Input: dimensioned drawing with shaded views. Units: mm. Origin: part minimum x, y, z. Round coordinates to 2 decimals unless told otherwise and drop trailing zeros. Write each loop counter-clockwise with the first axis right and the second up, starting at its lowest first coordinate (ties: lowest second). Pieces come first, ordered by that corner, then holes. Notation, with made-up numbers: (48, 53.25) - (105, 53.25) arc R31 cw to (105, 91.25) - close; hole circle Ø8 at (75, 69). An arc over 180 degrees is marked (long way). Use one line per item in the form item = value.
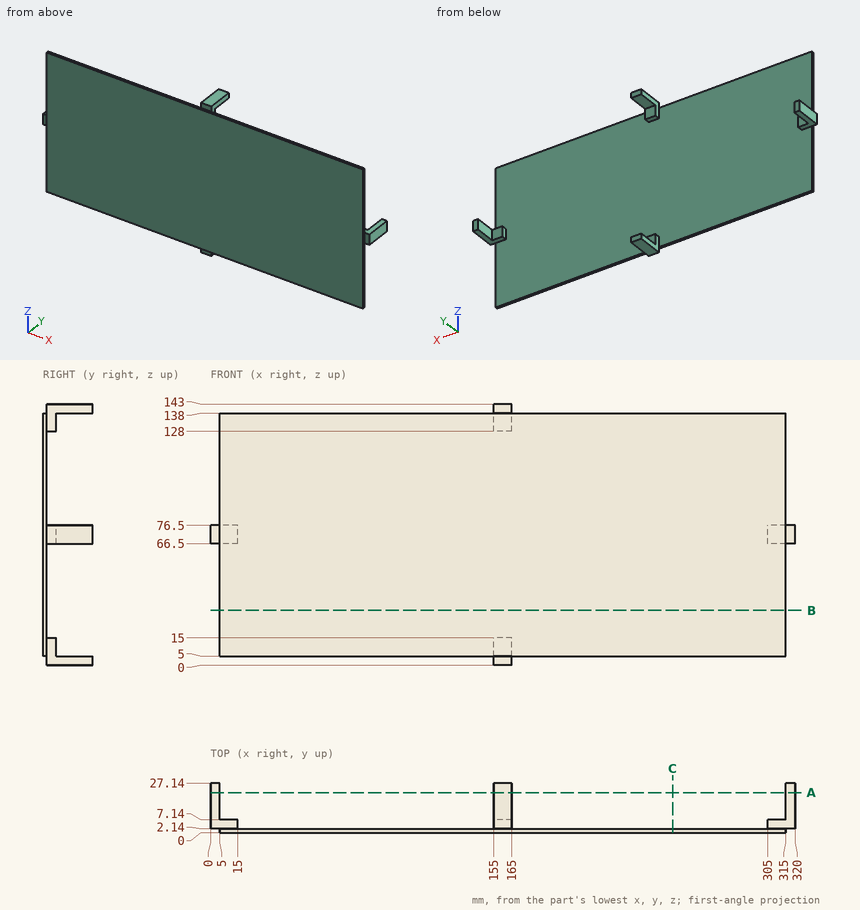
(1) Cut plane B-B on z = 30. Output: boundary loops of the cut face in (x, y).
Derived:
outline = (5, 0) - (315, 0) - (315, 2.14) - (5, 2.14) - close
(2) Cut plane C-C on x = 253. Output: boundary loops of the cut face in (y, z).
Derived:
outline = (0, 5) - (2.14, 5) - (2.14, 138) - (0, 138) - close
(3) Material intervals for L1, parallel to X at y = 6.25, z = 73; L2, parallel to Z at x = 159, y = 25.75; L3, parallel to Y at x = 74.5, z = 98, sorted ascending.
Derived:
L1 = 0 to 15, 305 to 320
L2 = 0 to 5, 138 to 143
L3 = 0 to 2.14
(4) First-contact query: pin 1 Ø10 at (x, z) = (175.5, 75) entering from +Y; pin 2 Ø7.5 at (y, z) = (16.5, 5.5) entering from +X; pin 3 Ø2.5 at (y, z) = (1.5, 84.5) entering from +X; pin 4 Ø4.5 at (x, y) = (311.5, 12) entering from -Z. Flat tips, straight axial feed; report the tip coordinate or a pass-through.
Derived:
pin_1 = 2.14
pin_2 = 165
pin_3 = 315
pin_4 = through
(5) Cut plane A-A on y = 22. Output: boundary loops of the cut face in (x, z).
Derived:
outline = (0, 66.5) - (5, 66.5) - (5, 76.5) - (0, 76.5) - close; (155, 0) - (165, 0) - (165, 5) - (155, 5) - close; (155, 138) - (165, 138) - (165, 143) - (155, 143) - close; (315, 66.5) - (320, 66.5) - (320, 76.5) - (315, 76.5) - close
